from build123d import *

# Parameters (mm, degrees)
SKETCH1_W           = 38.1
SKETCH1_H           = 76.2
SKETCH1_R           = 1.8288
SKETCH1_R_2         = 6.35
BOSS_EXTRUDE1_DEPTH = 5.08
SKETCH2_W           = 5.08
SKETCH2_H           = 10.16
SKETCH2_W_2         = 7.62
SKETCH2_H_2         = 5.08
CUT_EXTRUDE1_DEPTH  = 5.08


with BuildPart() as part:
    # Sketch1 → Boss-Extrude1 (new body)
    with BuildSketch(Plane(origin=(0, 0, 0), x_dir=(0, 0, -1), z_dir=(1, 0, 0))):
        with Locations((-19.05, -9.087068966)):
            Rectangle(SKETCH1_W, SKETCH1_H)
        with Locations((-19.05, -18.358068966)):
            Circle(SKETCH1_R, mode=Mode.SUBTRACT)
        with Locations((-19.05, -28.137068966)):
            Circle(SKETCH1_R_2, mode=Mode.SUBTRACT)
        with Locations((-12.135202787, -21.222271752)):
            Circle(SKETCH1_R, mode=Mode.SUBTRACT)
        with Locations((-9.271, -28.137068966)):
            Circle(SKETCH1_R, mode=Mode.SUBTRACT)
        with Locations((-12.135202787, -35.051866179)):
            Circle(SKETCH1_R, mode=Mode.SUBTRACT)
        with Locations((-19.05, -37.916068966)):
            Circle(SKETCH1_R, mode=Mode.SUBTRACT)
        with Locations((-25.964797213, -35.051866179)):
            Circle(SKETCH1_R, mode=Mode.SUBTRACT)
        with Locations((-28.829, -28.137068966)):
            Circle(SKETCH1_R, mode=Mode.SUBTRACT)
        with Locations((-25.964797213, -21.222271752)):
            Circle(SKETCH1_R, mode=Mode.SUBTRACT)
    extrude(amount=BOSS_EXTRUDE1_DEPTH)

    # Sketch2 → Cut-Extrude1 (cut)
    with BuildSketch(Plane(origin=(5.08, 0, 0), x_dir=(0, 0, -1), z_dir=(1, 0, 0))):
        with Locations((-30.48, 23.932931034)):
            Rectangle(SKETCH2_W, SKETCH2_H)
        with Locations((-7.62, 23.932931034)):
            Rectangle(SKETCH2_W, SKETCH2_H)
        with Locations((-19.05, 23.932931034)):
            Rectangle(SKETCH2_W_2, SKETCH2_H)
        with Locations((-30.48, -6.547068966)):
            Rectangle(SKETCH2_W, SKETCH2_H_2)
        with Locations((-19.05, -6.547068966)):
            Rectangle(SKETCH2_W_2, SKETCH2_H_2)
        with Locations((-7.62, -6.547068966)):
            Rectangle(SKETCH2_W, SKETCH2_H_2)
    extrude(amount=-CUT_EXTRUDE1_DEPTH, mode=Mode.SUBTRACT)


solid = part.part
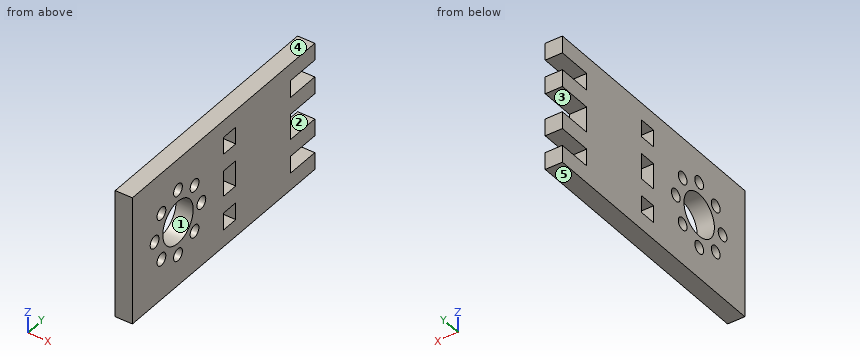
Model file for the job. Use its own axes, mm. Face numbers are marked on the shaded views. A direction names the side the tool comes from. Coordinates: 2 decimals unless noted, no trailing zeros. Order: outer loops, then holes, each group sorted by start corner. A loop starts at its lowest first (then second) coordinate and runs counter-clockwise, first axis right, second up. Notation, with made-up numbers: M -29,74.25 L -21,74.25 A25 ccw -21,86.25 Z; hole C 89,-29 d7. An arc over 180 degrees is marked long. Return JSON: item names as keys, results as strings.
1. Tool access for the marked faces 1 and 2: list every direction of +Z, -Z, +X, -X, +Y, -Y with a clear straight run to the whole face (end or side of a thin tool).
Ans:
{"face 1": "+X, -X", "face 2": "+X, -X, +Y"}
2. Flat gauge pins, fed straight in: pin 1 (8 mm diameter, centred on y = -15.5, z = 29.5, fed in from -X); pin 2 (2.5 mm diameter, centred on x = 1.5, z = 8.5, fed in from +Y). Where does each tip first touch, or does it go through?
Ans:
{"pin 1": "x = 0", "pin 2": "y = 18.85"}
3. Saw through at C-C (x = 3.5). Give the number of separate pieces and of enclosed holes in the cut face, and give its area (3 significant figures).
Ans:
{"separate pieces": "1", "enclosed holes": "12", "area": "2,420 mm^2"}
4. Drill centre lines: probe 1 along Z at (x, y) = (4.25, -6); probe 2 along Y at (x, z) = (2.4, 19.05); probe 3 along Y at (x, z) = (4.5, 31.5). Where is each one in solid material? Low to high.
Ans:
{"probe 1": "0 to 5.08, 10.16 to 15.24, 22.86 to 27.94, 33.02 to 38.1", "probe 2": "-47.19 to -39.74, -36.09 to -34.49, -21.79 to -20.19, -16.53 to -9.09, -4.01 to 18.85", "probe 3": "-47.19 to -9.09, -4.01 to 18.85"}
5. Saw through at A-A (z = 19.05). Give the cut face in (x, y).
Ans:
{"outline": "M 0,-47.19 L 5.08,-47.19 L 5.08,-39.74 L 0,-39.74 Z; M 0,-36.09 L 5.08,-36.09 L 5.08,-34.49 L 0,-34.49 Z; M 0,-21.79 L 5.08,-21.79 L 5.08,-20.19 L 0,-20.19 Z; M 0,-16.53 L 5.08,-16.53 L 5.08,-9.09 L 0,-9.09 Z; M 0,-4.01 L 5.08,-4.01 L 5.08,18.85 L 0,18.85 Z"}
6. Pull direction Z, two halves, no side cores. Call the marked faces 3, 4 and 5: +Z half, -Z half, draft (parallel to the pull), parting line (faces both ways), or undercut.
Ans:
{"face 3": "undercut", "face 4": "+Z half", "face 5": "-Z half"}
7. Saw through at B-B (z = 29). Give the cut face in (x, y).
Ans:
{"outline": "M 0,-47.19 L 5.08,-47.19 L 5.08,-29.96 L 0,-29.96 Z; M 0,-26.32 L 5.08,-26.32 L 5.08,-9.09 L 0,-9.09 Z; M 0,-4.01 L 5.08,-4.01 L 5.08,18.85 L 0,18.85 Z"}
